Job drawing, mm, ordinate dimensions from the low corner. One solid piece. Give positions to 0.01 mm unless a question says otherwise; leave off trailing zeros. Order: outer loops, then holes, each group sorted by start corner. A loop starts at its lowest first (then second) coordinate and runs counter-clockwise, first axis right, second up. Notation, with made-up numbers: (51, 54.25) - (89, 54.25) arc R17 ccw to (89, 71.25) - close; hole circle Ø6 at (-27.75, 83.5). An arc over 180 degrees is marked (long way). Use one line per item in the form item = value. Start each with the question number.
1. Band-saw the part on C-C, the plane x = 91.5. List the corners of the cut face in (y, z).
2. Drill centre lines: line 1 (Y direction, x = 84, z = 5.9); line 2 (X direction, y = 58, z = 5.25); line 3 (Y direction, x = 91.5, z = 2.25). Where is each one in solid material? Low to high.
3. Band-saw the part on A-A, the plane z = 5. List the corners of the cut face in (x, y).
4. Pull direction X, two halves, no side cores. Call the marked faces 1 and 2: +X half, -X half, draft (parallel to the pull), parting line (faces both ways), or undercut.
5. Band-saw the part on D-D, the plane y = 10.5. List the corners of the cut face in (x, z).
6. Pin check, flat tips, straight feed: P1, Ø1.4, axis at x = 11.5, y = 11, coming from the +Z side; P2, Ø4, axis at x = 91.5, y = 65.5, coming from the +Z side. Stop position of each tip, or through.
7. Band-saw the part on B-B, the plane y = 65.5. List the corners of the cut face in (x, z).
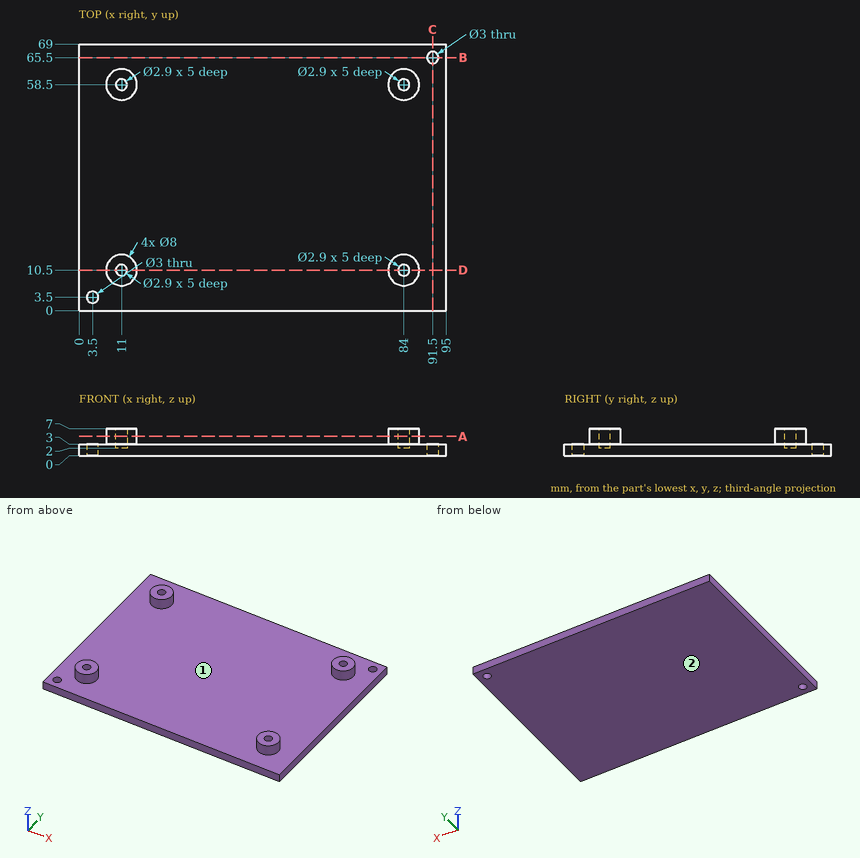
From the geometry:
q1.outline = (0, 0) - (64, 0) - (64, 3) - (0, 3) - close; (67, 0) - (69, 0) - (69, 3) - (67, 3) - close
q2.line_1 = 6.5 to 9.05, 11.95 to 14.5, 54.5 to 57.05, 59.95 to 62.5
q2.line_2 = 7.03 to 9.64, 12.36 to 14.97, 80.03 to 82.64, 85.36 to 87.97
q2.line_3 = 0 to 64, 67 to 69
q3.outline = circle Ø8 at (11, 10.5); circle Ø8 at (11, 58.5); circle Ø8 at (84, 10.5); circle Ø8 at (84, 58.5); hole circle Ø2.9 at (11, 10.5); hole circle Ø2.9 at (11, 58.5); hole circle Ø2.9 at (84, 10.5); hole circle Ø2.9 at (84, 58.5)
q4.face_1 = undercut
q4.face_2 = draft
q5.outline = (0, 0) - (95, 0) - (95, 3) - (88, 3) - (88, 7) - (85.45, 7) - (85.45, 2) - (82.55, 2) - (82.55, 7) - (80, 7) - (80, 3) - (15, 3) - (15, 7) - (12.45, 7) - (12.45, 2) - (9.55, 2) - (9.55, 7) - (7, 7) - (7, 3) - (0, 3) - close
q6.P1 = 2
q6.P2 = 3
q7.outline = (0, 0) - (90, 0) - (90, 3) - (0, 3) - close; (93, 0) - (95, 0) - (95, 3) - (93, 3) - close
